Work out the finished part from the listing and answer in its coordinate system (mm). A direction names the side the tool comes from. Give positions to 0.01 mm unless a question says otherwise; leave off trailing zeros. Write item = value, one per line. Start each with the question number.
1. Flat-ended cylindrical pins translate along their axes: pin 1 Ø3 at (x, z) = (27, -3) entering from +Y; pin 2 Ø1 at (x, z) = (-24.5, -1.5) entering from -Y; pin 3 Ø8 at (x, y) = (-52.5, -90.93) entering from -Z; pin 4 Ø1.5 at (x, z) = (-2, -2.5) entering from -Y. Find the tip coordinate at first contact, or state that the pin passes through.
2. For faces 1 (the face through (-2, 90, 0)), 2 (the face through (12.11, 89.51, -2.46)), determine the directions among +Z, -Z, +X, -X, +Y, -Y from which every point of the face is accessible in a straight line to the end or side of a thin tool.
3. The mould has two halves that part along X. Classify faces 3 (the face through (71.231, 111.725, -2.465)), 4 (the face through (-2, 90, -5)), 5 (the face through (-53.91, 75.166, -2.465)): released by +X, released by -X, zero draft, split by the parting line, or undercut.
4. Consider L1, parallel to Y at x = -32.5, z = -4.55; L2, parallel to X at y = 78, z = -1; L3, parallel to Y at x = 81, z = -3.5. Determine where each line is inside the solid, lowest interval first. Write a range as [from, to].
5. Section A-A on z = -0.85 is taken. Give the number of separate pieces and of enclosed holes in the cut face, plus the area to 3 significant figures.
Autodesk Inventor part; units mm, degrees
ref_plane "YZ Plane" through (0, 0, 0) normal (1, 0, 0) x (0, 1, 0)
ref_plane "XZ Plane" through (0, 0, 0) normal (0, 1, 0) x (-1, 0, 0)
ref_plane "XY Plane" through (0, 0, 0) normal (0, 0, 1) x (1, 0, 0)
sketch "Skizze1" plane through (0, 0, 0) normal (0, 0, 1) x (1, 0, 0)
  circle A0 centre (0, 0) radius 132.5
  line L0 (-185.5, 0) -> (185.5, 0)
  line L1 (0, -185.5) -> (0, 185.5)
  circle A1 centre (0, 0) radius 80 construction
  circle A2 centre (0, 80) radius 4
  line L2 (8.2396, 71.7385) -> (9.3594, 84.538)
  line L3 (-8.2396, 71.7385) -> (-9.3594, 84.538)
  line L4 (-5.251, 69) -> (5.251, 69)
  arc A3 (-9.3594, 84.538) -> (-17.4836, 90.8327) centre (-16.3328, 83.9279) ccw
  arc A4 (17.4836, 90.8327) -> (9.3594, 84.538) centre (16.3328, 83.9279) ccw
  arc A5 (-8.2396, 71.7385) -> (-5.251, 69) centre (-5.251, 72) ccw
  arc A6 (5.251, 69) -> (8.2396, 71.7385) centre (5.251, 72) ccw
  circle A7 centre (-76.0845, 24.7214) radius 4
  line L5 (-65.6812, 30.0047) -> (-77.5082, 35.025)
  line L6 (-70.7736, 14.3321) -> (-83.2926, 17.2224)
  line L7 (-67.2455, 16.3282) -> (-64.0002, 26.3162)
  arc A8 (-83.2926, 17.2224) -> (-91.7897, 11.441) centre (-84.8673, 10.4018) ccw
  arc A9 (-80.9843, 44.6967) -> (-77.5082, 35.025) centre (-74.7731, 41.4685) ccw
  arc A10 (-70.7736, 14.3321) -> (-67.2455, 16.3282) centre (-70.0987, 17.2552) ccw
  arc A11 (-64.0002, 26.3162) -> (-65.6812, 30.0047) centre (-66.8534, 27.2432) ccw
  circle A12 centre (-47.0228, -64.7214) radius 4
  line L8 (-48.8328, -53.1946) -> (-57.2621, -62.8914)
  line L9 (-35.5009, -62.8808) -> (-42.1183, -73.894)
  line L10 (-36.309, -58.9086) -> (-44.8053, -52.7357)
  arc A13 (-42.1183, -73.894) -> (-39.2456, -83.7618) centre (-36.1181, -77.4993) ccw
  arc A14 (-67.5346, -63.2086) -> (-57.2621, -62.8914) centre (-62.5451, -58.299) ccw
  arc A15 (-35.5009, -62.8808) -> (-36.309, -58.9086) centre (-38.0724, -61.3357) ccw
  arc A16 (-44.8053, -52.7357) -> (-48.8328, -53.1946) centre (-46.5687, -55.1628) ccw
  circle A17 centre (47.0228, -64.7214) radius 4
  line L11 (35.5009, -62.8808) -> (42.1183, -73.894)
  line L12 (48.8328, -53.1946) -> (57.2621, -62.8914)
  line L13 (44.8053, -52.7357) -> (36.309, -58.9086)
  arc A18 (57.2621, -62.8914) -> (67.5346, -63.2086) centre (62.5451, -58.299) ccw
  arc A19 (39.2456, -83.7618) -> (42.1183, -73.894) centre (36.1181, -77.4993) ccw
  arc A20 (48.8328, -53.1946) -> (44.8053, -52.7357) centre (46.5687, -55.1628) ccw
  arc A21 (36.309, -58.9086) -> (35.5009, -62.8808) centre (38.0724, -61.3357) ccw
  circle A22 centre (76.0845, 24.7214) radius 4
  line L14 (70.7736, 14.3321) -> (83.2926, 17.2224)
  line L15 (65.6812, 30.0047) -> (77.5082, 35.025)
  line L16 (64.0002, 26.3162) -> (67.2455, 16.3282)
  arc A23 (77.5082, 35.025) -> (80.9843, 44.6967) centre (74.7731, 41.4685) ccw
  arc A24 (91.7897, 11.441) -> (83.2926, 17.2224) centre (84.8673, 10.4018) ccw
  arc A25 (65.6812, 30.0047) -> (64.0002, 26.3162) centre (66.8534, 27.2432) ccw
  arc A26 (67.2455, 16.3282) -> (70.7736, 14.3321) centre (70.0987, 17.2552) ccw
  arc A27 (80.9843, 44.6967) -> (17.4836, 90.8327) centre (0, 0) ccw
  arc A28 (-17.4836, 90.8327) -> (-80.9843, 44.6967) centre (0, 0) ccw
  arc A29 (-91.7897, 11.441) -> (-67.5346, -63.2086) centre (0, 0) ccw
  arc A30 (-39.2456, -83.7618) -> (39.2456, -83.7618) centre (0, 0) ccw
  arc A31 (67.5346, -63.2086) -> (91.7897, 11.441) centre (0, 0) ccw
  point P0 (10.0088, 91.9605)
  point P1 (-10.0088, 91.9605)
  point P2 (-8, 69)
  point P3 (8, 69)
  point P4 (-68.095, 13.7137)
  point P5 (-63.1508, 28.9306)
  point P6 (-34.085, -60.5245)
  point P7 (-47.0293, -51.1199)
  point P8 (47.0293, -51.1199)
  point P9 (34.085, -60.5245)
  point P10 (63.1508, 28.9306)
  point P11 (68.095, 13.7137)
  dimension "d2" = 160
  dimension "d0" = 265
  dimension "d3" = 8
  dimension "d5" = 10
  dimension "d6" = 16
  dimension "d7" = 7
  dimension "d8" = 3
  dimension "d11" = 360
  dimension "d36" = 69
extrude "Extrusion1" add sketch "Skizze1" against normal blind 5 contours L0 A31 A24 L14 A26 L16 A25 L15 A23 A27 A4 L2 A6 L4 L1 A2 A0 | A0 L1 A30 A19 L11 A21 L13 A20 L12 A18 A31 L0 | L1 A2 L4 A5 L3 A3 A28 A9 L5 A11 L7 A10 L6 A8 A29 L0 A0 | A0 L0 A29 A14 L8 A16 L10 A15 L9 A13 A30 L1
sketch "Skizze2" plane through (0, 0, 0) normal (0, 0, 1) x (1, 0, 0)
  line L0 (-185.5, 0) -> (185.5, 0) construction
  line L1 (0, -185.5) -> (0, 185.5) construction
  circle A0 centre (0, 105) radius 2.5
  circle A1 centre (15, 112.5) radius 2.5
  circle A2 centre (32, 115) radius 2.5
  dimension "d23" = 5
  dimension "d24" = 5
  dimension "d25" = 5
  dimension "d26" = 105
  dimension "d27" = 112.5
  dimension "d28" = 115
  dimension "d29" = 15
  dimension "d30" = 32
extrude "Extrusion2" cut sketch "Skizze2" against normal through all
pattern_circular "Runde Anordnung1" count 12 over 360 about axis through (0, 0, -10) along (0, 0, 1) of "Extrusion2"
properties part number "HP2 Raceparts 002" material "钢，高强度，低合金"
Verdict:
q1.pin_1 = 130.02
q1.pin_2 = -130.31
q1.pin_3 = -5
q1.pin_4 = -132.49
q2.face_1 = +Z, +X, -X, +Y, -Y
q2.face_2 = +Z, -Z
q3.face_3 = split by the parting line
q3.face_4 = zero draft
q3.face_5 = undercut
q4.L1 = [-128.45, -117.45], [-112.55, -86.6], [86.6, 128.45]
q4.L2 = [-107.11, -49.72], [-8.79, -3.46], [3.46, 8.79], [49.72, 107.11]
q4.L3 = [-104.86, -44.67], [16.69, 38.27], [44.67, 104.86]
q5.separate_pieces = 1
q5.enclosed_holes = 42
q5.area = 29,500 mm2
